Read the model definition and answer for the solid it produces. Units are mm, in the model's axes. A direction names the side the tool comes from. Give positions to 0.01 mm unless a question says otherwise; leave off trailing zeros. Loops run counter-clockwise (first coordinate to the right, second up) from the corner with the lowest first, then second, coordinate; pieces in that order, holes last. Notation, with made-up numbers: (87, 49) - (100, 49) arc R19 ccw to (100, 82) - close; hole circle Ø8 at (-9.75, -0.5). An arc over 180 degrees is marked (long way). Write item = value, one per line. Start each with the question number.
from build123d import *

# Parameters (mm, degrees)
EXTRUDE_1_DEPTH      = 6
SKETCH_2_W           = 5
SKETCH_2_H           = 22
EXTRUDE_2_DEPTH      = 31
CHAMFER_1_SIZE       = 6
SKETCH_3_W           = 12
SKETCH_3_H           = 8
CUT_EXTRUDE_1_DEPTH  = 57.73623181
SKETCH_4_W           = 3
SKETCH_4_H           = 21
CUT_EXTRUDE_2_DEPTH  = 60.110066825
MIRROR_START         = 13
MIRROR_1_DEPTH       = 22
MIRROR_START_2       = -35
MIRROR_1_2_OUTLINE_W = 16
MIRROR_1_2_OUTLINE_H = 3
MIRROR_1_2_DEPTH     = 57
MIRROR_1_3_OUTLINE_W = 16
MIRROR_1_3_OUTLINE_H = 3
MIRROR_1_3_DEPTH     = 17
MIRROR_START_3       = 3
MIRROR_1_4_OUTLINE_W = 16
MIRROR_1_4_OUTLINE_H = 3
MIRROR_1_4_DEPTH     = 19


# Read off the part's stored shape, not the designer's step: the mirror step
with BuildPart() as part:
    # Sketch 1 → Extrude 1 (new body)
    with BuildSketch(Plane.XY):
        Polygon((-15, 22), (-15, -35), (1, -35), (1, 13), (15, 13), (15, 35), (-10, 35), (-10, 22), align=None)
    extrude(amount=EXTRUDE_1_DEPTH)

    # Sketch 2 → Extrude 2 (add)
    with BuildSketch(Plane.XY.offset(6)):
        with Locations((12.5, 24)):
            Rectangle(SKETCH_2_W, SKETCH_2_H)
    extrude(amount=EXTRUDE_2_DEPTH)

    # Chamfer 1
    chamfer_1_edges = [part.edges().sort_by_distance(p)[0] for p in [
        (15, 24, 0),
    ]]
    chamfer(chamfer_1_edges, length=CHAMFER_1_SIZE)

    # Sketch 3 → Cut-Extrude 1 (cut, through all)
    with BuildSketch(Plane.ZY.offset(-10)):
        with Locations((24, 24)):
            Rectangle(SKETCH_3_W, SKETCH_3_H)
    extrude(amount=-CUT_EXTRUDE_1_DEPTH, mode=Mode.SUBTRACT)

    # Sketch 4 → Cut-Extrude 2 (cut, through all)
    with BuildSketch(Plane.ZY.offset(15)):
        with Locations((1.5, -7.5)):
            Rectangle(SKETCH_4_W, SKETCH_4_H)
    extrude(amount=-CUT_EXTRUDE_2_DEPTH, mode=Mode.SUBTRACT)



with BuildPart() as body_2:
    # Mirror 1 outline → Mirror 1 (new body)
    with BuildSketch(Plane(origin=(0, 0, 0), x_dir=(1, 0, 0), z_dir=(0, 1, 0)).offset(MIRROR_START)):
        Polygon((-40, -6), (-20, -6), (-20, 0), (-39, 0), (-45, -6), (-45, -37), (-40, -37), align=None)
    extrude(amount=MIRROR_1_DEPTH)


with BuildPart() as part_1:
    add(part.part)

    add(body_2.part)  # Mirror 1 2 merges body 2
    # Mirror 1 2 outline → Mirror 1 2 (add)
    with BuildSketch(Plane(origin=(0, 0, 0), x_dir=(1, 0, 0), z_dir=(0, 1, 0)).offset(MIRROR_START_2)):
        with Locations((-23, -4.5)):
            Rectangle(MIRROR_1_2_OUTLINE_W, MIRROR_1_2_OUTLINE_H)
    extrude(amount=MIRROR_1_2_DEPTH)

    # Mirror 1 3 outline → Mirror 1 3 (add)
    with BuildSketch(Plane(origin=(0, 0, 0), x_dir=(1, 0, 0), z_dir=(0, 1, 0)).offset(MIRROR_START_2)):
        with Locations((-23, -1.5)):
            Rectangle(MIRROR_1_3_OUTLINE_W, MIRROR_1_3_OUTLINE_H)
    extrude(amount=MIRROR_1_3_DEPTH)

    # Mirror 1 4 outline → Mirror 1 4 (add)
    with BuildSketch(Plane(origin=(0, 0, 0), x_dir=(1, 0, 0), z_dir=(0, 1, 0)).offset(MIRROR_START_3)):
        with Locations((-23, -1.5)):
            Rectangle(MIRROR_1_4_OUTLINE_W, MIRROR_1_4_OUTLINE_H)
    extrude(amount=MIRROR_1_4_DEPTH)


solid = part_1.part
1. A tool of negligible diameter and unlimited length cuts with its end or side. For faces 1 (the flat face through (-20, 28, 3)), 2 (the flat face through (11, 13, 14)), 3 (the flat face through (-31, -11, 4)), 4 (the flat face through (12, 20, 24)), 5 (the flat face through (-15, 7, 6)), from which of +Z, -Z, +X, -X, +Y, -Y can it reach the whole face along a straight path? Write none if from no direction.
2. Given P1, Ø6.5, axis at y = 31.5, z = 2.5, coming from the -X side; P2, Ø6.5, axis at y = -18, z = 3, coming from the -X side; P3, Ø5, axis at y = -21, z = 2.5, coming from the +X side; P4, Ø12, axis at x = 2, z = 24.5, coming from the +Y side, each flat-ended and moving along its own axis, determine where each tip first touches the part or whether it passes through.
3. A cutting plane is placed at B-B on x = -21.5. Give the vertices of the cut face in (y, z), and give its area (3 significant figures).
4. A cutting plane is placed at C-C on y = -12. Give the vertices of the cut face in (x, z).
5. A cutting plane is placed at A-A on z = 17. Give the vertices of the cut face in (x, y), and give its area (3 significant figures).
6. For a pull along Y with two mould halves and no side action, classify faces 6 (the flat face through (12, 28, 24)), 7 (the flat face through (-41, 13, 14)), 8 (the flat face through (12, 24, 30)), 9 (the flat face through (-15, 22, 3)) as released by +Y, released by -Y, zero draft, split by the parting line, or undercut.
7. Consider line 1 along X through (y, z) = (32, 14); line 2 along X through (y, z) = (0, 4.5); line 3 along Z through (x, y) = (-27, 1.5). Determine where each line is inside the solid, lowest interval first. Write a range as [from, to].
8. A cutting plane is placed at D-D on x = -14. Give the vertices of the cut face in (y, z), and give its area (3 significant figures).
Reply:
q1.face_1 = +Z, -Z, +Y
q1.face_2 = +Z, -Z, +X, -Y
q1.face_3 = +Z, -Z, -X, -Y
q1.face_4 = +X
q1.face_5 = +Z, +Y, -Y
q2.P1 = -44.75
q2.P2 = -31
q2.P3 = 1
q2.P4 = through
q3.outline = (-35, 0) - (-18, 0) - (-18, 3) - (3, 3) - (3, 0) - (35, 0) - (35, 6) - (-35, 6) - close
q3.area = 357 mm^2
q4.outline = (-31, 3) - (1, 3) - (1, 6) - (-31, 6) - close
q5.outline = (-45, 13) - (-40, 13) - (-40, 35) - (-45, 35) - close; (10, 13) - (15, 13) - (15, 35) - (10, 35) - close
q5.area = 220 mm^2
q6.face_6 = undercut
q6.face_7 = released by -Y
q6.face_8 = undercut
q6.face_9 = released by +Y
q7.line_1 = [-45, -40], [10, 15]
q7.line_2 = [-31, 1]
q7.line_3 = [3, 6]
q8.outline = (-35, 0) - (-18, 0) - (-18, 3) - (3, 3) - (3, 0) - (22, 0) - (22, 6) - (-35, 6) - close
q8.area = 279 mm^2
